CAD build for the part. Positions are in the model's coordinates, mm. A direction names the side the tool comes from. Round coordinates to 2 decimals unless told otherwise and drop trailing zeros. Order: outer loops, then holes, each group sorted by start corner. A loop starts at its lowest first (then second) coordinate and runs counter-clockwise, first axis right, second up. Notation, with made-up numbers: (0, 41) - (15, 41) arc R20 ccw to (15, 73) - close; hole circle Ø10 at (-28, 12.5). An arc over 180 degrees is marked (long way). Write item = value, one per line.
from build123d import *

# Parameters (mm, degrees)
SKETCH_1_W          = 10
SKETCH_1_H          = 18
EXTRUDE_1_DEPTH     = 2
SKETCH_2_R          = 2.25
CUT_EXTRUDE_1_DEPTH = 2
EXTRUDE_2_DEPTH     = 3
CHAMFER_1_SIZE      = 1
EXTRUDE_START       = -18
EXTRUDE_3_DEPTH     = 3
FILLET_1_R          = 2


with BuildPart() as part:
    # Эскиз1 → Бобышка-Вытянуть1 (new body)
    with BuildSketch(Plane(origin=(0, 0, 0), x_dir=(1, 0, 0), z_dir=(0, 1, 0))):
        with Locations((5, 9)):
            Rectangle(SKETCH_1_W, SKETCH_1_H)
    extrude(amount=EXTRUDE_1_DEPTH)

    # Эскиз2 → Вырез-Вытянуть1 (cut)
    with BuildSketch(Plane(origin=(0, 2, 0), x_dir=(1, 0, 0), z_dir=(0, 1, 0))):
        with Locations(Location((5, 9, 0), (0, 0, 270))):
            Circle(SKETCH_2_R)
    extrude(amount=-CUT_EXTRUDE_1_DEPTH, mode=Mode.SUBTRACT)

    # Эскиз4 → Бобышка-Вытянуть2 (add)
    with BuildSketch(Plane.XY):
        with BuildLine():
            Line((0, 6), (0, 2))
            Line((0, 2), (2, 2))
            Line((2, 2), (2, 4))
            ThreePointArc((2, 4), (2.292893219, 4.707106781), (3, 5))
            Line((3, 5), (7, 5))
            ThreePointArc((7, 5), (7.707106781, 4.707106781), (8, 4))
            Line((8, 4), (8, 2))
            Line((8, 2), (10, 2))
            Line((10, 2), (10, 6))
            ThreePointArc((10, 6), (9.707106781, 6.707106781), (9, 7))
            Line((9, 7), (8, 7))
            Line((8, 7), (2, 7))
            Line((2, 7), (1, 7))
            ThreePointArc((1, 7), (0.292893219, 6.707106781), (0, 6))
        make_face()
    extrude(amount=-EXTRUDE_2_DEPTH)

    # Фаска1
    chamfer_1_edges = [part.edges().sort_by_distance(p)[0] for p in [
        (5, 2, -11.25),
    ]]
    chamfer(chamfer_1_edges, length=CHAMFER_1_SIZE)

    # Эскиз4<3> → Бобышка-Вытянуть3 (add)
    with BuildSketch(Plane.XY.offset(EXTRUDE_START)):
        with BuildLine():
            Line((0, 2), (2, 2))
            Line((2, 2), (2, 4))
            ThreePointArc((2, 4), (2.292893219, 4.707106781), (3, 5))
            Line((3, 5), (7, 5))
            ThreePointArc((7, 5), (7.707106781, 4.707106781), (8, 4))
            Line((8, 4), (8, 2))
            Line((8, 2), (10, 2))
            Line((10, 2), (10, 6))
            ThreePointArc((10, 6), (9.707106781, 6.707106781), (9, 7))
            Line((9, 7), (8, 7))
            Line((8, 7), (2, 7))
            Line((2, 7), (1, 7))
            ThreePointArc((1, 7), (0.292893219, 6.707106781), (0, 6))
            Line((0, 6), (0, 2))
        make_face()
    extrude(amount=EXTRUDE_3_DEPTH)

    # Скругление1
    fillet_1_edges = [part.edges().sort_by_distance(p)[0] for p in [
        (9, 2, -3),
        (1, 2, -3),
        (1, 2, -15),
        (9, 2, -15),
    ]]
    fillet(fillet_1_edges, radius=FILLET_1_R)


solid = part.part
(1) Band-saw the part on B-B on y = 1.5. List the corners of the cut face in (x, z), plus the area to 3 significant figures.
Solved:
outline = (0, -18) - (10, -18) - (10, 0) - (0, 0) - close; hole circle Ø5.5 at (5, -9)
area = 156 mm²
(2) Pull direction X, two halves, no side cores. Call faces 1 (the flat face through (2, 3, -16)), 2 (the flat face through (5, 6, -15)), 3 (the flat face through (0, 1.7, -8.9)): released by +X, released by -X, zero draft, split by the parting line, or undercut.
Solved:
face_1 = undercut
face_2 = zero draft
face_3 = released by -X
(3) Band-saw the part on A-A on z = -9. List the corners of the cut face in (x, y).
Solved:
outline = (0, 0) - (2.75, 0) - (2.75, 1) - (1.75, 2) - (0, 2) - close; (7.25, 0) - (10, 0) - (10, 2) - (8.25, 2) - (7.25, 1) - close
(4) Tool access for faces 4 (the flat face through (1.6, 2, -9.1)), 5 (the cylindrical face through (9.715, 6.699, -16.521)), 6 (the cylindrical face through (9.01, 2.6, -3.57)), 7 (the flat face through (10, 1.6, -8.9)), 8 (the cylindrical face through (7.699, 4.715, -1.479)): list every direction of +Z, -Z, +X, -X, +Y, -Y with a clear straight run to the whole face (end or side of a thin tool).
Solved:
face_4 = none
face_5 = +Z, -Z, +X, +Y
face_6 = +X, -X, +Y
face_7 = +Z, -Z, +X, +Y, -Y
face_8 = +Z, -Z
(5) Probe line 1 along Z through (x, y) = (9, 5.75); line 2 along X through (y, z) = (0.3, -9); line 3 along Y through (x, z) = (7, -2.5). List the from-to ranges inside material, lowest first.
Solved:
line_1 = -18 to -15, -3 to 0
line_2 = 0 to 2.75, 7.25 to 10
line_3 = 0 to 2, 5 to 7
(6) Drop flat-ended pins along their axis: pin 1 (2.5 mm diameter, centred on x = 5, z = -9, fed in from -Y); pin 2 (3 mm diameter, centred on x = 4, z = -6, fed in from +Y). Give the stop position or say it passes through.
Solved:
pin_1 = through
pin_2 = 2
(7) Band-saw the part on D-D on y = 3. List the corners of the cut face in (x, z).
Solved:
outline = (0, -18) - (2, -18) - (2, -14.73) - (0, -14.73) - close; (0, -3.27) - (2, -3.27) - (2, 0) - (0, 0) - close; (8, -18) - (10, -18) - (10, -14.73) - (8, -14.73) - close; (8, -3.27) - (10, -3.27) - (10, 0) - (8, 0) - close
(8) Band-saw the part on C-C on x = 5. List the corners of the cut face in (y, z), plus the area to 3 significant figures.
Solved:
outline = (0, -18) - (2, -18) - (2, -12.25) - (1, -11.25) - (0, -11.25) - close; (0, -6.75) - (1, -6.75) - (2, -5.75) - (2, 0) - (0, 0) - close; (5, -18) - (7, -18) - (7, -15) - (5, -15) - close; (5, -3) - (7, -3) - (7, 0) - (5, 0) - close
area = 38.0 mm²
